Check sheet for the drawn part. Datum: minimum x, y, z corner. Units: mm. Give positions to 0.01 mm unless a question says otherwise; leave off trailing zeros. Loops run counter-clockwise (first coordinate to the right, second up) from the corner with the lowest first, then second, coordinate; pieces in that order, holes last. Notation, with made-up numbers: (83, -2.75) - (89, -2.75) arc R5 cw to (89, 4.25) - close; hole circle Ø9 at (79.5, 16). An arc over 180 degrees is marked (long way). One line per item, written item: value. Start each with the question number.
1. Sectioned sample at C-C (y = 76). Record the cut outline in (x, z), plus the area to 3 significant figures.
2. Mould release check, pull along Y, two halves, no side actions. Record for the marked faces 1, 2 and 3: pulls with the +Y half, pulls with the -Y half, needs draft (parallel to the pull), parting line crosses it, or undercut.
3. Scan lines: L1, parallel to Z at x = 10, y = 98.5; L2, parallel to Z at x = 24.5, y = 631 (1 decimal). Record each from-to range of solid material in increasing order. Write a range as [from, to].
4. Sectioned sample at B-B (x = 31.5). Record the cut outline in (y, z), plus the area to 4 significant figures.
5. Sectioned sample at A-A (z = 76.5). Record the cut outline in (x, y), plus the area to 3 significant figures.
6. Gauge pin test, flat end, axial feed: pin 1 (13.5 mm diameter, centred on x = 19, y = 519, fed in from +Z). Record the tip position at first contact, or that the pin passes through.
7. Sectioned sample at D-D (z = 26.5). Record the cut outline in (x, y) (1 decimal), plus the area to 3 significant figures.
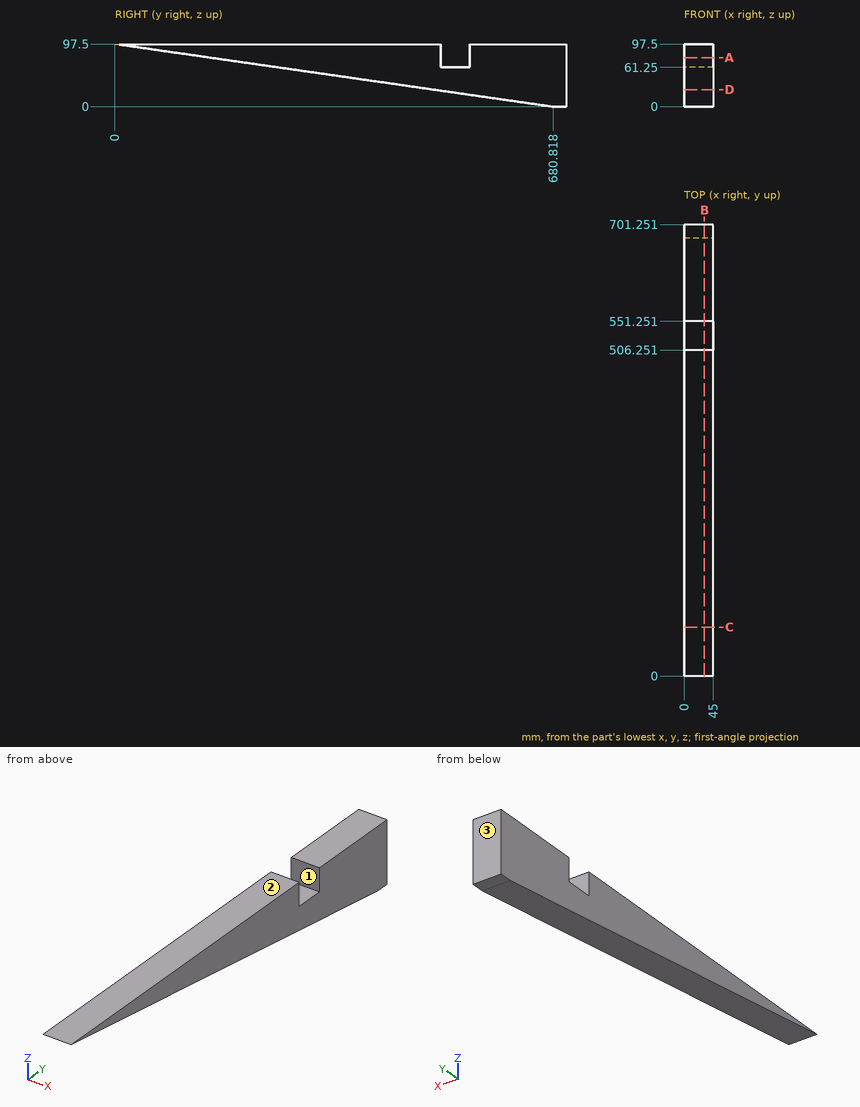
Results are:
1. outline: (0, 86.62) - (45, 86.62) - (45, 97.5) - (0, 97.5) - close
1. area: 490 mm^2
2. face 1: undercut
2. face 2: needs draft
2. face 3: pulls with the +Y half
3. L1: z = [83.39, 97.5]
3. L2: z = [7.1, 97.5]
4. outline: (0, 97.5) - (680.82, 0) - (701.25, 0) - (701.25, 97.5) - (551.25, 97.5) - (551.25, 61.25) - (506.25, 61.25) - (506.25, 97.5) - close
4. area: 33,550 mm^2
5. outline: (0, 146.64) - (45, 146.64) - (45, 506.25) - (0, 506.25) - close; (0, 551.25) - (45, 551.25) - (45, 701.25) - (0, 701.25) - close
5. area: 22,900 mm^2
6. pin 1: stops at z = 61.25
7. outline: (0, 495.8) - (45, 495.8) - (45, 701.3) - (0, 701.3) - close
7. area: 9,250 mm^2
